For this review, take the finished solid that the model builds, in its own axes (mm). Face numbers are marked on the shaded views. A direction names the side the tool comes from. Give positions to 0.01 mm unless a question says otherwise; leave off trailing zeros. Order: outer loops, then holes, each group sorted by start corner. A loop starts at its lowest first (then second) coordinate and runs counter-clockwise, first axis right, second up. Notation, with made-up numbers: (80, 15.5) -> (124, 15.5) arc R28 cw to (124, 42.5) -> close; hole circle Ø3 at (68.25, 20.5). An arc over 180 degrees is marked (long way). Return JSON: item names as keys, results as strings. Group by question number.
1) Add section C-C (y = 17). Give the boundary of the cut face in (x, z).
2) The part is to be moulded in two halves that separate along X. For the marked faces 1, 2, 3 and 4, say which applies: released by +X, released by -X, zero draft, split by the parting line, or undercut.
3) Insertion check: P1, Ø9, axis at x = 27, y = 26.5, coming from the +Z side; P2, Ø3, axis at x = 46.5, z = 26.5, coming from the -Y side; P3, Ø5.5, axis at x = 128, y = 10, coming from the +Z side. Each pin has a flat end and moves straight along its axis. Give the tip position at first contact, or say it passes through.
4) Add section A-A (x = 17). Give the boundary of the cut face in (y, z).
5) To check wall thickness, follow line 1 along Y through (x, z) = (17, 3); line 2 along X through (y, z) = (11.5, 14); line 3 along Z through (x, y) = (29, 25.5). State the ranges of each line that lie inside material, in increasing order.
6) For the marked faces 5, 6 and 7, list the 3-axis set-ups (+Z, -Z, +X, -X, +Y, -Y) from which the entire face can be reached by the end or side of a thin tool; tool diameter is ignored.
7) Add section B-B (z = 25.5). State how many separate pieces and enclosed holes the cut face has, then the cut area to 3 significant figures.
from build123d import *

# Parameters (mm, degrees)
ESQUISSE1_W                  = 140
ESQUISSE1_H                  = 40
BOSS_EXTRU_1_DEPTH           = 30
ESQUISSE2_W                  = 30
ESQUISSE2_H                  = 40
ENL_V_MAT_EXTRU_1_DEPTH      = 20
ENL_V_MAT_EXTRU_2_DEPTH      = 149.660687473
ENL_V_MAT_EXTRU_2_DEPTH_BACK = 149.660687473
ENL_V_MAT_EXTRU_6_DEPTH      = 149.660687473
ENL_V_MAT_EXTRU_6_DEPTH_BACK = 149.660687473
ESQUISSE5_R                  = 3
CONG_1_R                     = 10
ESQUISSE6_W                  = 30
ESQUISSE6_H                  = 5
BOSS_EXTRU_2_DEPTH           = 30
CONG_2_R                     = 4
CONG_3_R                     = 2
CONG_4_R                     = 5


with BuildPart() as part:
    # Esquisse1 → Boss.-Extru.1 (new body)
    with BuildSketch(Plane.XY):
        with Locations((70, 20)):
            Rectangle(ESQUISSE1_W, ESQUISSE1_H)
    extrude(amount=BOSS_EXTRU_1_DEPTH)

    # Esquisse2 → Enlèv. mat.-Extru.1 (cut)
    with BuildSketch(Plane.XY.offset(30)):
        with Locations((25, 20)):
            Rectangle(ESQUISSE2_W, ESQUISSE2_H)
    extrude(amount=-ENL_V_MAT_EXTRU_1_DEPTH, mode=Mode.SUBTRACT)

    # Esquisse3 → Enlèv. mat.-Extru.2 (cut, two sides: drawn at the far end of the back side and taken through both)
    with BuildSketch(Plane.XY.offset(30).offset(-ENL_V_MAT_EXTRU_2_DEPTH_BACK)):
        Polygon((140, 20), (60, 40), (140, 40), align=None)
    extrude(amount=ENL_V_MAT_EXTRU_2_DEPTH + ENL_V_MAT_EXTRU_2_DEPTH_BACK, mode=Mode.SUBTRACT)

    # Esquisse5 → Enlèv. mat.-Extru.6 (cut, two sides: drawn at the far end of the back side and taken through both)
    with BuildSketch(Plane.XY.offset(30).offset(-ENL_V_MAT_EXTRU_6_DEPTH_BACK)):
        with Locations(Location((17, 32, 0), (0, 0, 180))):
            Circle(ESQUISSE5_R)
        with Locations(Location((33, 8, 0), (0, 0, 180))):
            Circle(ESQUISSE5_R)
        with Locations(Location((68, 22, 0), (0, 0, 180))):
            Circle(ESQUISSE5_R)
        with Locations(Location((128, 10, 0), (0, 0, 180))):
            Circle(ESQUISSE5_R)
    extrude(amount=ENL_V_MAT_EXTRU_6_DEPTH + ENL_V_MAT_EXTRU_6_DEPTH_BACK, mode=Mode.SUBTRACT)

    # Congé1
    cong_1_edges = [part.edges().sort_by_distance(p)[0] for p in [
        (140, 20, 15),
    ]]
    fillet(cong_1_edges, radius=CONG_1_R)

    # Esquisse6 → Boss.-Extru.2 (add)
    with BuildSketch(Plane.XY.offset(30)):
        with Locations((125, -2.5)):
            Rectangle(ESQUISSE6_W, ESQUISSE6_H)
    extrude(amount=-BOSS_EXTRU_2_DEPTH)

    # Congé2
    cong_2_edges = [part.edges().sort_by_distance(p)[0] for p in [
        (110, 0, 15),
    ]]
    fillet(cong_2_edges, radius=CONG_2_R)

    # Congé3
    cong_3_edges = [part.edges().sort_by_distance(p)[0] for p in [
        (140, -5, 15),
        (110, -5, 15),
    ]]
    fillet(cong_3_edges, radius=CONG_3_R)

    # Congé4
    cong_4_edges = [part.edges().sort_by_distance(p)[0] for p in [
        (0, 40, 15),
        (0, 0, 15),
    ]]
    fillet(cong_4_edges, radius=CONG_4_R)


solid = part.part
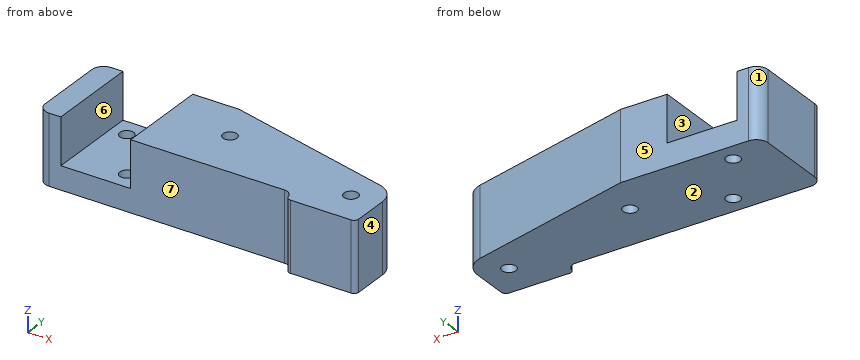
Evaluation:
{
 "1": {"outline": "(0, 0) -> (138.77, 0) -> (138.77, 30) -> (40, 30) -> (40, 10) -> (10, 10) -> (10, 30) -> (0, 30) -> close"},
 "2": {"face 1": "released by -X", "face 2": "zero draft", "face 3": "undercut", "face 4": "released by +X"},
 "3": {"P1": "z = 10", "P2": "y = 0", "P3": "through"},
 "4": {"outline": "(0, 0) -> (29, 0) -> (29, 10) -> (0, 10) -> close; (35, 0) -> (40, 0) -> (40, 10) -> (35, 10) -> close"},
 "5": {"line 1": "0 to 29, 35 to 40", "line 2": "0 to 10, 40 to 125.4, 130.6 to 140", "line 3": "0 to 10"},
 "6": {"face 5": "+Z, -Z, +X, -X, +Y", "face 6": "+Z, +Y, -Y", "face 7": "+Z, -Z, -X, -Y"},
 "7": {"separate pieces": "2", "enclosed holes": "2", "area": "3,670 mm^2"}
}
